from build123d import *

# Parameters (mm, degrees)
F0_R      = 13.5
F1_DEPTH  = 3.25
F3_R      = 4.25
F1_FACE_R = 13.5
F5_R      = 4.25
F6_DEPTH  = 7.5


with BuildPart() as f1:
    # F0 (on Front) → F1 (new body)
    with BuildSketch(Plane.XZ):
        Circle(F0_R)
    extrude(amount=F1_DEPTH)

    # F3 (on offset) → F4 section 0
    with BuildSketch(Plane.XZ.offset(11)):
        Circle(F3_R)
    # F1_face (on face) → F4 section 1
    with BuildSketch(Plane.XZ.offset(3.25)):
        Circle(F1_FACE_R)
    loft()

    # F5 (on face) → F6 (cut)
    with BuildSketch(Plane.XZ.offset(11)):
        Circle(F5_R)
    extrude(amount=-F6_DEPTH, mode=Mode.SUBTRACT)


solid = f1.part
Verification items for the finished model (mm, model axes). Coordinates: 2 decimals unless noted, no trailing zeros. Loops run counter-clockwise (first coordinate to the right, second up) from the corner with the lowest first, then second, coordinate; pieces in that order, holes last. Notation, with made-up numbers: M 23.25,-25 L 82.25,-25 A33 cw 82.25,14 Z; hole C 33,-21 d8. An arc over 180 degrees is marked long. One line per item, written item: value.
1. Mould release check, pull along X, two halves, no side actions. Record for faces 1 (the flat face through (0, -3.5, 0)), 2 (the flat face through (0, 0, 0)), 3 (the cylindrical face through (-2.93, -1.6, -13.18)), 4 (the cylindrical face through (2.285, -7.302, 3.584)): pulls with the +X half, pulls with the -X half, needs draft (parallel to the pull), parting line crosses it, or undercut.
Answers follow:
face 1: undercut
face 2: needs draft
face 3: parting line crosses it
face 4: undercut
2. Gauge pin test, flat ends, axial feed: P1, Ø1, axis at y = -5, z = -1.5, coming from the -X side; P2, Ø1.5, axis at x = -6.5, z = -8.5, coming from the -Y side; P3, Ø4, axis at x = -2, z = -0.5, coming from the -Y side. Record the tip position at first contact, or that the pin passes through.
Answers follow:
P1: x = -11.92
P2: y = -6.22
P3: y = -3.5
3. Section check C-C on y = -4.25. Record the cut outline in (x, z), plus the area to 3 significant figures.
Answers follow:
outline: C 0,0 d24.61; hole C 0,0 d8.5
area: 419 mm^2
4. Section check D-D on y = -7. Record the cut outline in (x, z).
Answers follow:
outline: C 0,0 d18.05; hole C 0,0 d8.5
5. Section check A-A on x = 0. Record the cut outline in (y, z), plus the area to 3 significant figures.
Answers follow:
outline: M -11,-4.25 L -3.25,-13.5 L 0,-13.5 L 0,13.5 L -3.25,13.5 L -11,4.25 L -3.5,4.25 L -3.5,-4.25 Z
area: 162 mm^2
6. Material ranges on line 1 along Z through (x, y) = (0, -5.75); line 2 along X through (y, z) = (-10.5, 2.75); line 3 along Z through (x, y) = (0, -7.25), recorded low to high. Write a range as from..to.
Answers follow:
line 1: -10.52..-4.25, 4.25..10.52
line 2: -3.99..-3.24, 3.24..3.99
line 3: -8.73..-4.25, 4.25..8.73
7. Section check B-B on y = -2. Record the cut outline in (x, z).
Answers follow:
outline: C 0,0 d27
